The model under review builds one solid part; all positions refer to its coordinate system, in mm. Coordinates: 2 decimals unless noted, no trailing zeros. Order: outer loops, then holes, each group sorted by start corner. A loop starts at its lowest first (then second) coordinate and runs counter-clockwise, first axis right, second up. Notation, with made-up numbers: (5, -10) -> (9, -10) arc R19 cw to (9, 11) -> close; hole circle Ø3 at (17, 8.25). An arc over 180 degrees is marked (long way). Use one line per item in the form item = value. Start each with the question number.
(1) Wall thickness on line 1 along Y through (x, z) = (22.75, 4.25); line 2 along X through (y, z) = (3.25, 8); line 3 along X through (y, z) = (12.5, 6.5): over which ranges is each line inside the solid? List them lowest first.
(2) Take a section at B-B (y = 13). State the section outline as (x, z) points, then the cut area to 3 significant figures.
(3) Insertion check: pin 1 Ø4 at (x, z) = (4, 3) entering from +Y; pin 2 Ø3 at (y, z) = (10.5, 5.5) entering from -X; pin 3 Ø1 at (x, z) = (26, 6) entering from +Y. Each pin has a flat end and moves straight along its axis. Give the tip position at first contact, or say it passes through.
(4) Take a section at C-C (x = 6). State the section outline as (y, z) points.
```python
from build123d import *

# Parameters (mm, degrees)
SKETCH1_W           = 30
SKETCH1_H           = 15
BOSS_EXTRUDE1_DEPTH = 10
FILLET1_R           = 7.5


with BuildPart() as part:
    # Sketch1 → Boss-Extrude1 (new body)
    with BuildSketch(Plane.XY):
        with Locations((15, 7.5)):
            Rectangle(SKETCH1_W, SKETCH1_H)
    extrude(amount=BOSS_EXTRUDE1_DEPTH)

    # Fillet1
    fillet1_edges = [part.edges().sort_by_distance(p)[0] for p in [
        (30, 0, 5),
        (30, 15, 5),
        (0, 0, 5),
        (0, 15, 5),
    ]]
    fillet(fillet1_edges, radius=FILLET1_R - 0.0001)  # a hair under: the kernel refuses the full size


solid = part.part
```
Findings:
q1.line_1 = 0 to 15
q1.line_2 = 1.32 to 28.68
q1.line_3 = 1.91 to 28.09
q2.outline = (2.4, 0) -> (27.6, 0) -> (27.6, 10) -> (2.4, 10) -> close
q2.area = 252 mm²
q3.pin_1 = 14.85
q3.pin_2 = 0.15
q3.pin_3 = 14.37
q4.outline = (0.15, 0) -> (14.85, 0) -> (14.85, 10) -> (0.15, 10) -> close
